```python
from build123d import *

# Parameters (mm, degrees)
SKETCH1_W            = 8
SKETCH1_H            = 24
BOSS_EXTRUDE1_DEPTH  = 9.6
SKETCH2_R            = 2.4
BOSS_EXTRUDE2_DEPTH  = 1.6
LPATTERN1_COUNT      = 2
LPATTERN1_PITCH      = 8
LPATTERN1_COUNT_DIR2 = 4
LPATTERN1_PITCH_DIR2 = 8
SHELL1_T             = -1.6


with BuildPart() as part:
    # Sketch1 → Boss-Extrude1 (new body)
    with BuildSketch(Plane(origin=(0, 0, 0), x_dir=(1, 0, 0), z_dir=(0, 1, 0))):
        with Locations((4, 12)):
            Rectangle(SKETCH1_W, SKETCH1_H)
    extrude(amount=BOSS_EXTRUDE1_DEPTH)

    # Sketch2 → Boss-Extrude2 (add)
    with BuildSketch(Plane(origin=(0, 9.6, 0), x_dir=(1, 0, 0), z_dir=(0, 1, 0))):
        with Locations(Location((4, 4, 0), (0, 0, 90))):
            Circle(SKETCH2_R)
    boss_extrude2 = extrude(amount=BOSS_EXTRUDE2_DEPTH)

    # LPattern1: Boss-Extrude2 2 × 4, 5 skipped
    with Locations(*[(i * LPATTERN1_PITCH, 0, -j * LPATTERN1_PITCH_DIR2) for i in range(LPATTERN1_COUNT) for j in range(LPATTERN1_COUNT_DIR2) if (i, j) not in ((0, 0), (0, 3), (1, 0), (1, 1), (1, 2), (1, 3))]):
        add(boss_extrude2)

    # Shell1
    shell1_openings = [part.faces().sort_by_distance(p)[0] for p in [
        (4, 0, -12),
    ]]
    offset(amount=SHELL1_T, openings=shell1_openings, kind=Kind.INTERSECTION)


solid = part.part
```
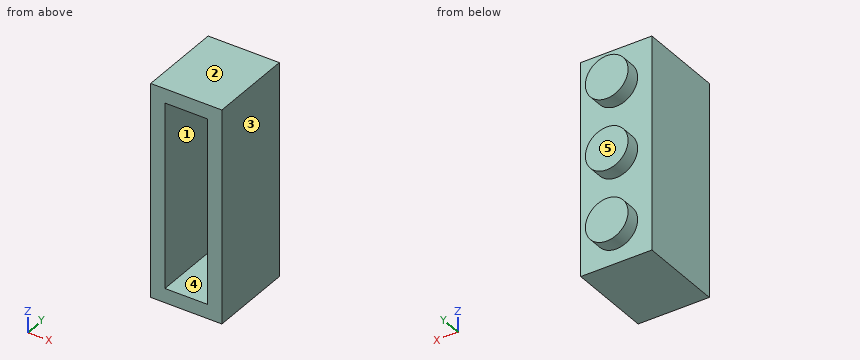
Geometry check sheet. Reference: the model listing, model coordinates, mm. Face numbers are marked on the shaded views. A direction names the side the tool comes from. Give positions to 0.01 mm unless a question says otherwise; leave off trailing zeros. Write each loop counter-clockwise with the first axis right and the second up, starting at its lowest first coordinate (ties: lowest second). Pieces come first, ordered by that corner, then holes. Notation, with made-up numbers: (77.25, 32) -> (91.25, 32) arc R15 ccw to (91.25, 37) -> close; hole circle Ø3 at (3.5, -22). An arc over 180 degrees is marked (long way). Use one line per item in the form item = value.
Item 1: Mould release check, pull along X, two halves, no side actions. Record for the marked faces 3, 4 and 5: released by +X, released by -X, zero draft, split by the parting line, or undercut.
Results list:
face_3 = released by +X
face_4 = undercut
face_5 = zero draft
Item 2: Sectioned sample at B-B on z = -20. Enter the section's corners in (x, y).
Results list:
outline = (0, 0) -> (1.6, 0) -> (1.6, 8) -> (3.2, 8) -> (3.2, 9.6) -> (4.8, 9.6) -> (4.8, 8) -> (6.4, 8) -> (6.4, 0) -> (8, 0) -> (8, 9.6) -> (6.4, 9.6) -> (6.4, 11.2) -> (1.6, 11.2) -> (1.6, 9.6) -> (0, 9.6) -> close
Item 3: Depth check by flat-ended pin: pin 1 Ø3 at (x, y) = (2, 9) entering from +Z; pin 2 Ø1.3 at (x, z) = (3.5, -4) entering from -Y. Enter the tip coordinate at first touch or a pass-through.
Results list:
pin_1 = 0
pin_2 = 8
Item 4: Scan lines: line 1 (X direction, y = 9.1, z = -12); line 2 (X direction, y = 4, z = -3.25); line 3 (Z direction, x = 4, y = 6.75). Record each from-to range of solid material in increasing order.
Results list:
line_1 = 0 to 3.2, 4.8 to 8
line_2 = 0 to 1.6, 6.4 to 8
line_3 = -24 to -22.4, -1.6 to 0
Item 5: Sectioned sample at C-C on y = 8.5. Enter the section's corners in (x, z), plus the area to 3 significant figures.
Results list:
outline = (0, -24) -> (8, -24) -> (8, 0) -> (0, 0) -> close; hole circle Ø1.6 at (4, -20); hole circle Ø1.6 at (4, -12); hole circle Ø1.6 at (4, -4)
area = 186 mm2
Item 6: Sectioned sample at A-A on y = 6. Enter the section's corners in (x, z), plus the area to 3 significant figures.
Results list:
outline = (0, -24) -> (8, -24) -> (8, 0) -> (0, 0) -> close; hole (1.6, -22.4) -> (6.4, -22.4) -> (6.4, -1.6) -> (1.6, -1.6) -> close
area = 92.2 mm2
Item 7: Sectioned sample at D-D on y = 10. Enter the section's corners in (x, z).
Results list:
outline = circle Ø4.8 at (4, -20); circle Ø4.8 at (4, -12); circle Ø4.8 at (4, -4)
Item 8: Access from +Z, -Z, +X, -X, +Y, -Y to the whole of each face (thin tool, end or side, straight path). Record for the marked faces 1 and 2.
Results list:
face_1 = -Y
face_2 = +Z, +X, -X, +Y, -Y
